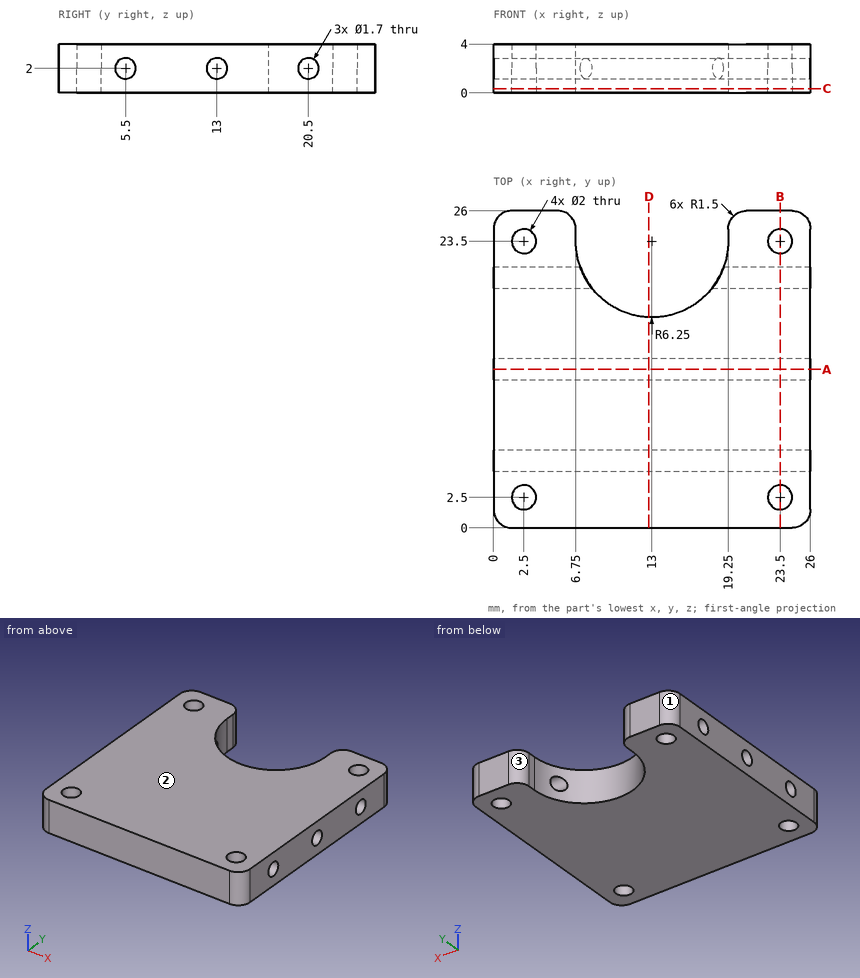
Check sheet for the drawn part. Datum: minimum x, y, z corner. Units: mm. Round coordinates to 2 decimals unless told otherwise and drop trailing zeros. Loops run counter-clockwise (first coordinate to the right, second up) from the corner with the lowest first, then second, coordinate; pieces in that order, holes last. Notation, with made-up numbers: (12, 29) - (27, 29) arc R7 cw to (27, 34) - close; hole circle Ø2 at (13, -29.5). An arc over 180 degrees is marked (long way). Write item = value, one per line. Start each with the question number.
1. Section check B-B on x = 23.5. Enter the section's corners in (y, z), then the cut area to 3 significant figures.
2. Thickness scan on line 1 (Y direction, x = 17, z = 1.9); line 2 (Z direction, x = 4, y = 20.5); line 3 (Y direction, x = 9.75, z = 1.55). Record the ranges inside material, lowest first.
3. Section check A-A on y = 13. Enter the section's corners in (x, z).
4. Mould release check, pull along X, two halves, no side actions. Record for the marked faces 1, 2 and 3: released by +X, released by -X, zero draft, split by the parting line, or undercut.
5. Depth check by flat-ended pin: pin 1 (3 mm diameter, centred on x = 23.5, y = 23.5, fed in from -Z); pin 2 (1.2 mm diameter, centred on x = 2.5, y = 2.5, fed in from -Z). Enter the tip coordinate at first touch or a pass-through.
6. Section check C-C on z = 0.35. Enter the section's corners in (x, y).
7. Section check D-D on x = 12.75. Enter the section's corners in (y, z) (3 decimals), then the cut area to 3 significant figures.
Working result:
q1.outline = (0, 0) - (1.5, 0) - (1.5, 4) - (0, 4) - close; (3.5, 0) - (22.5, 0) - (22.5, 4) - (3.5, 4) - close; (24.5, 0) - (26, 0) - (26, 4) - (24.5, 4) - close; hole circle Ø1.7 at (5.5, 2); hole circle Ø1.7 at (13, 2); hole circle Ø1.7 at (20.5, 2)
q1.area = 81.2 mm^2
q2.line_1 = 0 to 4.66, 6.34 to 12.16, 13.84 to 18.7
q2.line_2 = 0 to 1.15, 2.85 to 4
q2.line_3 = 0 to 4.78, 6.22 to 12.28, 13.72 to 18.16
q3.outline = (0, 0) - (26, 0) - (26, 1.15) - (0, 1.15) - close; (0, 2.85) - (26, 2.85) - (26, 4) - (0, 4) - close
q4.face_1 = released by -X
q4.face_2 = zero draft
q4.face_3 = undercut
q5.pin_1 = 0
q5.pin_2 = through
q6.outline = (0, 1.5) arc R1.5 ccw to (1.5, 0) - (24.5, 0) arc R1.5 ccw to (26, 1.5) - (26, 24.5) arc R1.5 ccw to (24.5, 26) - (20.75, 26) arc R1.5 ccw to (19.25, 24.5) - (19.25, 23.5) arc R6.25 cw to (6.75, 23.5) - (6.75, 24.5) arc R1.5 ccw to (5.25, 26) - (1.5, 26) arc R1.5 ccw to (0, 24.5) - close; hole circle Ø2 at (2.5, 2.5); hole circle Ø2 at (2.5, 23.5); hole circle Ø2 at (23.5, 2.5); hole circle Ø2 at (23.5, 23.5)
q7.outline = (0, 0) - (17.255, 0) - (17.255, 4) - (0, 4) - close; hole circle Ø1.7 at (5.5, 2); hole circle Ø1.7 at (13, 2)
q7.area = 64.5 mm^2
